Input: part model. Units: mm. Frame: model coordinates. A direction names the side the tool comes from. Coordinates: 2 decimals unless noted, no trailing zeros. Write each loop counter-clockwise with the first axis right and the second up, starting at its lowest first coordinate (ties: lowest second). Pieces come first, ordered by that corner, then holes. Notation, with made-up numbers: (-31.75, -29) -> (20.25, -29) arc R22 cw to (20.25, -22) -> close; hole circle Ø10 at (74.25, 64). An arc over 180 degrees is marked (long way). Use one line per item in the form item = value. Start each with the question number.
(1) Cut plane C-C on x = 0. Return the cut outline in (y, z), plus the area to 3 significant figures.
(2) Ray query, line 1 along Y through (x, z) = (-17, 0); line 2 along Y through (x, z) = (31, -12.5); line 3 along Y through (x, z) = (16, 0). Return the intervals inside material, ascending.
(3) Cut plane A-A on y = 0. Return the cut outline in (x, z).
(4) Pull-direction query (Z, two-part tool) for faces 6 (the face through (-29.335, 91.776, -0.187)), 7 (the face through (26.335, 92, 15)), 8 (the face through (-17.535, -1.341, 3.233)); classes: released by +Z, released by -Z, zero draft, split by the parting line, or undercut.
(5) Set-up query: faces 1 (the face through (21, 36, 0)), 2 (the face through (-20, 3, 6)), 3 (the face through (-0.438, 91.776, 31.332)), 4 (the face through (-27.238, 110.145, -15.348)), 5 (the face through (-3.417, 115.465, -0.759)). Return all of +Z, -Z, +X, -X, +Y, -Y with unobstructed straight access to the full face (end or side cutting, diameter ignored); none if empty.
(6) First-contact query: pin 1 (3.5 mm diameter, centred on y = -1.5, z = 0.5, fed in from +X); pin 2 (8 mm diameter, centred on x = -27.5, z = 1, fed in from +Y); pin 3 (11 mm diameter, centred on y = 0, z = 0, fed in from +X). Flat tips, straight axial feed; report the tip coordinate or a pass-through.
(7) Cut plane D-D on y = 97. Return the cut outline in (x, z), plus the area to 3 significant figures.
(8) Cut plane B-B on z = 0. Return the cut outline in (x, y), plus the area to 3 significant figures.
```python
from build123d import *
from build123d.topology import SkipClean

# Parameters (mm, degrees)
CUT_EXTRUDE1_DEPTH      = 35
CUT_EXTRUDE1_DEPTH_BACK = 35
SKETCH2_OUTSIDE_W       = 96.248
SKETCH2_OUTSIDE_H       = 96.248
BOSS_EXTRUDE1_DEPTH     = 36
SKETCH4_R               = 3.5
CUT_EXTRUDE2_DEPTH      = 5
LPATTERN1_COUNT         = 2
LPATTERN1_PITCH         = 35
BOSS_EXTRUDE2_DEPTH     = 40
BOSS_EXTRUDE2_DRAFT     = -9
BOSS_EXTRUDE6_DEPTH     = 35
SKETCH10_R              = 35
BOSS_EXTRUDE7_DEPTH     = 2
FILLET5_R               = 3
SKETCH11_R              = 3.5
BOSS_EXTRUDE8_DEPTH     = 5


with BuildPart() as part:
    # Sketch1 → Revolve2 (revolve)
    with BuildSketch(Plane(origin=(0, 0, 0), x_dir=(1, 0, 0), z_dir=(0, 1, 0))):
        with BuildLine():
            Line((0, 35), (0, -35))
            ThreePointArc((0, -35), (35, 0), (0, 35))
        make_face()
    revolve(axis=Axis((0, 0, -35), (0, 0, 1)))

    # Sketch2 outside → Cut-Extrude1 (cut, two sides: drawn at the far end of the back side and taken through both)
    with SkipClean():  # the faces are left unmerged after this step: merging them gives an invalid solid
        with BuildSketch(Plane(origin=(0, 0, 0), x_dir=(1, 0, 0), z_dir=(0, 1, 0)).offset(-CUT_EXTRUDE1_DEPTH_BACK)):
            Rectangle(SKETCH2_OUTSIDE_W, SKETCH2_OUTSIDE_H)
            with BuildLine():
                Line((-20, -28.722813233), (-20, 28.722813233))
                ThreePointArc((-20, 28.722813233), (0, 35), (20, 28.722813233))
                Line((20, 28.722813233), (20, -28.722813233))
                ThreePointArc((20, -28.722813233), (0, -35), (-20, -28.722813233))
            make_face(mode=Mode.SUBTRACT)
        extrude(amount=CUT_EXTRUDE1_DEPTH + CUT_EXTRUDE1_DEPTH_BACK, mode=Mode.SUBTRACT)

    # Sketch3 → Boss-Extrude1 (add)
    with BuildSketch(Plane(origin=(0, 0, 0), x_dir=(1, 0, 0), z_dir=(0, 1, 0))):
        with BuildLine():
            Line((-20, 15), (-20, -15))
            ThreePointArc((-20, -15), (0, -25), (20, -15))
            Line((20, -15), (20, 15))
            ThreePointArc((20, 15), (0, 25), (-20, 15))
        make_face()
    extrude(amount=BOSS_EXTRUDE1_DEPTH)

    # Sketch4 → Cut-Extrude2 (cut)
    with BuildSketch(Plane.ZY.offset(20)):
        Circle(SKETCH4_R)
    cut_extrude2 = extrude(amount=-CUT_EXTRUDE2_DEPTH, mode=Mode.SUBTRACT)

    # LPattern1: Cut-Extrude2 ×2
    with Locations(*[(i * LPATTERN1_PITCH, 0, 0) for i in range(1, LPATTERN1_COUNT)]):
        add(cut_extrude2, mode=Mode.SUBTRACT)


with BuildPart() as boss_extrude2_tool:
    # Sketch5 → Boss-Extrude2 (with draft: the straight prism first)
    with BuildSketch(Plane(origin=(0, 36, 0), x_dir=(1, 0, 0), z_dir=(0, 1, 0))):
        with BuildLine():
            Line((-20, 15), (-20, 11.357816692))
            ThreePointArc((-20, 11.357816692), (-23, 0), (-20, -11.357816692))
            Line((-20, -11.357816692), (-20, -15))
            ThreePointArc((-20, -15), (0, -25), (20, -15))
            Line((20, -15), (20, -11.357816692))
            ThreePointArc((20, -11.357816692), (23, 0), (20, 11.357816692))
            Line((20, 11.357816692), (20, 15))
            ThreePointArc((20, 15), (0, 25), (-20, 15))
        make_face()
    extrude(amount=BOSS_EXTRUDE2_DEPTH)
    # Boss-Extrude2: the draft: its side faces are tilted about the plane it starts from
    boss_extrude2_sides = [boss_extrude2_tool.faces().sort_by_distance(p)[0] for p in [
        (20, 56, -13.178908346),
        (0, 56, -25),
        (-20, 56, -13.178908346),
        (-23, 56, 0),
        (-20, 56, 13.178908346),
        (0, 56, 25),
        (20, 56, 13.178908346),
        (23, 56, 0),
    ]]
    draft(boss_extrude2_sides, Plane(origin=(0, 36, 0), x_dir=(1, 0, 0), z_dir=(0, 1, 0)), BOSS_EXTRUDE2_DRAFT)


with BuildPart() as part_1:
    add(part.part)

    # Boss-Extrude2: add boss_extrude2_tool
    add(boss_extrude2_tool.part)

    # Sketch9 → Boss-Extrude6 (add)
    with BuildSketch(Plane(origin=(0, 76, 0), x_dir=(1, 0, 0), z_dir=(0, 1, 0))):
        with BuildLine():
            Line((26.335377613, 12.923322548), (26.335377613, 16.980982779))
            ThreePointArc((26.335377613, 16.980982779), (0, 31.335377613), (-26.335377613, 16.980982779))
            Line((-26.335377613, 16.980982779), (-26.335377613, 12.923322548))
            ThreePointArc((-26.335377613, 12.923322548), (-29.335377613, 0), (-26.335377613, -12.923322548))
            Line((-26.335377613, -12.923322548), (-26.335377613, -16.980982779))
            ThreePointArc((-26.335377613, -16.980982779), (0, -31.335377613), (26.335377613, -16.980982779))
            Line((26.335377613, -16.980982779), (26.335377613, -12.923322548))
            ThreePointArc((26.335377613, -12.923322548), (29.335377613, 0), (26.335377613, 12.923322548))
        make_face()
    extrude(amount=BOSS_EXTRUDE6_DEPTH)

    # Sketch10 → Boss-Extrude7 (add)
    with BuildSketch(Plane(origin=(0, 111, 0), x_dir=(1, 0, 0), z_dir=(0, 1, 0))):
        with Locations(Location((0, 0, 0), (0, 0, 270))):
            Circle(SKETCH10_R)
    extrude(amount=BOSS_EXTRUDE7_DEPTH)

    # Fillet5
    fillet5_edges = [part_1.edges().sort_by_distance(p)[0] for p in [
        (29.335377613, 111, 0),
        (26.335377613, 111, -14.952152663),
        (0, 111, -31.335377613),
        (-26.335377613, 111, -14.952152663),
        (-29.335377613, 111, 0),
        (-26.335377613, 111, 14.952152663),
        (0, 111, 31.335377613),
        (26.335377613, 111, 14.952152663),
    ]]
    fillet(fillet5_edges, radius=FILLET5_R)

    # Sketch11 → Boss-Extrude8 (add)
    with BuildSketch(Plane(origin=(0, 113, 0), x_dir=(1, 0, 0), z_dir=(0, 1, 0))):
        with Locations(Location((0, 0, 0), (0, 0, 270))):
            Circle(SKETCH11_R)
    extrude(amount=BOSS_EXTRUDE8_DEPTH)


solid = part_1.part
```
Values:
q1.outline = (24.49, -25) -> (36, -25) -> (76, -31.34) -> (108, -31.34) arc R3 cw to (111, -34.34) -> (111, -35) -> (113, -35) -> (113, -3.5) -> (118, -3.5) -> (118, 3.5) -> (113, 3.5) -> (113, 35) -> (111, 35) -> (111, 34.34) arc R3 cw to (108, 31.34) -> (76, 31.34) -> (36, 25) -> (24.49, 25) arc R35 ccw (long way) to start
q1.area = 8,690 mm2
q2.line_1 = -30.59 to -3.5, 3.5 to 113
q2.line_2 = 111 to 113
q2.line_3 = -31.13 to -3.5, 3.5 to 113
q3.outline = (-20, -28.72) arc R35 ccw to (20, -28.72) -> (20, -3.5) -> (15, -3.5) -> (15, 3.5) -> (20, 3.5) -> (20, 28.72) arc R35 ccw to (-20, 28.72) -> (-20, 3.5) -> (-15, 3.5) -> (-15, -3.5) -> (-20, -3.5) -> close
q4.face_6 = split by the parting line
q4.face_7 = zero draft
q4.face_8 = undercut
q5.face_1 = +Z, -Z, +X, -Y
q5.face_2 = +Z, -Z, -X, -Y
q5.face_3 = +Z
q5.face_4 = -Z, -X, -Y
q5.face_5 = +Y
q6.pin_1 = 15
q6.pin_2 = 113
q6.pin_3 = 20
q7.outline = (-26.34, -16.98) arc R31.34 ccw to (26.34, -16.98) -> (26.34, -12.92) arc R29.34 ccw to (26.34, 12.92) -> (26.34, 16.98) arc R31.34 ccw to (-26.34, 16.98) -> (-26.34, 12.92) arc R29.34 ccw to (-26.34, -12.92) -> close
q7.area = 2,960 mm2
q8.outline = (-35, 111) -> (-32.34, 111) arc R3 cw to (-29.34, 108) -> (-29.34, 76) -> (-23, 36) -> (-20, 36) -> (-20, 3.5) -> (-15, 3.5) -> (-15, -3.5) -> (-20, -3.5) -> (-20, -28.72) arc R35 ccw to (20, -28.72) -> (20, -3.5) -> (15, -3.5) -> (15, 3.5) -> (20, 3.5) -> (20, 36) -> (23, 36) -> (29.34, 76) -> (29.34, 108) arc R3 cw to (32.34, 111) -> (35, 111) -> (35, 113) -> (3.5, 113) -> (3.5, 118) -> (-3.5, 118) -> (-3.5, 113) -> (-35, 113) -> close
q8.area = 7,020 mm2
